from build123d import *

# Parameters (mm, degrees)
SKETCH_1_R                = 2.5
EXTRUDE_1_DEPTH           = 25.88
EXTRUDE_START             = 3
SKETCH_2_R                = 1
EXTRUDE_2_DEPTH           = 2
CUT_EXTRUDE_1_DEPTH       = 4
CUT_EXTRUDE_START         = 21.88
CUT_EXTRUDE_2_DEPTH       = 4
SKETCH_6_R                = 0.25
CUT_EXTRUDE_3_DEPTH       = 0.25
CUT_EXTRUDE_START_2       = 4.25
SKETCH_7_R                = 0.25
CUT_EXTRUDE_4_DEPTH       = 0.25
EXTRUDE_START_2           = 8
SKETCH_17_R               = 3.5
EXTRUDE_5_DEPTH           = 9.88
SKETCH_18_R               = 1
CUT_EXTRUDE_11_DEPTH      = 10
CUT_EXTRUDE_START_3       = 15.88
SKETCH_19_R               = 1
CUT_EXTRUDE_12_DEPTH      = 10
CUT_EXTRUDE_13_DEPTH      = 2.5
CUT_EXTRUDE_13_DEPTH_BACK = 2.5
SKETCH_20_W               = 4
SKETCH_20_H               = 1.6
CUT_EXTRUDE_14_DEPTH      = 28.789825476
CUT_EXTRUDE_14_DEPTH_BACK = 28.789825476
SKETCH_21_W               = 1.5
SKETCH_21_H               = 9.88
SKETCH_22_W               = 4
SKETCH_22_H               = 1.5
CUT_EXTRUDE_15_DEPTH      = 28.789825476


with BuildPart() as part:
    # 草图1 → 凸台-拉伸1 (new body)
    with BuildSketch(Plane(origin=(0, 0, 0), x_dir=(1, 0, 0), z_dir=(0, 1, 0))):
        with Locations(Location((0, 0, 0), (0, 0, 270))):
            Circle(SKETCH_1_R)
    extrude(amount=EXTRUDE_1_DEPTH)

    # 草图2 → 凸台-拉伸2 (add)
    with BuildSketch(Plane(origin=(0, 0, 0), x_dir=(1, 0, 0), z_dir=(0, 1, 0)).offset(EXTRUDE_START)):
        with BuildLine():
            Line((0.166666667, 2.494438258), (7.633333333, 1.995550606))
            ThreePointArc((7.633333333, 1.995550606), (9.5, 0), (7.633333333, -1.995550606))
            Line((7.633333333, -1.995550606), (0.166666667, -2.494438258))
            ThreePointArc((0.166666667, -2.494438258), (-2.5, 0), (0.166666667, 2.494438258))
        make_face()
        with Locations(Location((7.5, 0, 0), (0, 0, 270))):
            Circle(SKETCH_2_R, mode=Mode.SUBTRACT)
    extrude(amount=EXTRUDE_2_DEPTH)

    # 草图3 → 切除-拉伸1 (cut)
    with BuildSketch(Plane(origin=(0, 0, 0), x_dir=(1, 0, 0), z_dir=(0, 1, 0))):
        with BuildLine():
            Line((-1.854049622, -0.75), (-0.75, -0.75))
            Line((-0.75, -0.75), (-0.75, -1.854049622))
            ThreePointArc((-0.75, -1.854049622), (0, -2), (0.75, -1.854049622))
            Line((0.75, -1.854049622), (0.75, -0.75))
            Line((0.75, -0.75), (1.854049622, -0.75))
            ThreePointArc((1.854049622, -0.75), (2, 0), (1.854049622, 0.75))
            Line((1.854049622, 0.75), (0.75, 0.75))
            Line((0.75, 0.75), (0.75, 1.854049622))
            ThreePointArc((0.75, 1.854049622), (0, 2), (-0.75, 1.854049622))
            Line((-0.75, 1.854049622), (-0.75, 0.75))
            Line((-0.75, 0.75), (-1.854049622, 0.75))
            ThreePointArc((-1.854049622, 0.75), (-2, 0), (-1.854049622, -0.75))
        make_face()
    extrude(amount=CUT_EXTRUDE_1_DEPTH, mode=Mode.SUBTRACT)

    # 草图5 → 切除-拉伸2 (cut)
    with BuildSketch(Plane(origin=(0, 0, 0), x_dir=(1, 0, 0), z_dir=(0, 1, 0)).offset(CUT_EXTRUDE_START)):
        with BuildLine():
            Line((1.854049622, 0.75), (0.75, 0.75))
            Line((0.75, 0.75), (0.75, 1.854049622))
            ThreePointArc((0.75, 1.854049622), (0, 2), (-0.75, 1.854049622))
            Line((-0.75, 1.854049622), (-0.75, 0.75))
            Line((-0.75, 0.75), (-1.854049622, 0.75))
            ThreePointArc((-1.854049622, 0.75), (-2, 0), (-1.854049622, -0.75))
            Line((-1.854049622, -0.75), (-0.75, -0.75))
            Line((-0.75, -0.75), (-0.75, -1.854049622))
            ThreePointArc((-0.75, -1.854049622), (0, -2), (0.75, -1.854049622))
            Line((0.75, -1.854049622), (0.75, -0.75))
            Line((0.75, -0.75), (1.854049622, -0.75))
            ThreePointArc((1.854049622, -0.75), (2, 0), (1.854049622, 0.75))
        make_face()
    extrude(amount=CUT_EXTRUDE_2_DEPTH, mode=Mode.SUBTRACT)

    # 草图6 → 切除-拉伸3 (cut)
    with BuildSketch(Plane(origin=(0, 0, 0), x_dir=(1, 0, 0), z_dir=(0, 1, 0)).offset(CUT_EXTRUDE_START)):
        with Locations(Location((0.75, 0, 0), (0, 0, 270))):
            Circle(SKETCH_6_R)
    extrude(amount=-CUT_EXTRUDE_3_DEPTH, mode=Mode.SUBTRACT)

    # 草图7 → 切除-拉伸4 (cut)
    with BuildSketch(Plane(origin=(0, 0, 0), x_dir=(1, 0, 0), z_dir=(0, 1, 0)).offset(CUT_EXTRUDE_START_2)):
        with Locations(Location((0.75, 0, 0), (0, 0, 270))):
            Circle(SKETCH_7_R)
    extrude(amount=-CUT_EXTRUDE_4_DEPTH, mode=Mode.SUBTRACT)

    # 草图17 → 凸台-拉伸5 (add)
    with BuildSketch(Plane(origin=(0, 0, 0), x_dir=(1, 0, 0), z_dir=(0, 1, 0)).offset(EXTRUDE_START_2)):
        with Locations(Location((0, 0, 0), (0, 0, 270))):
            Circle(SKETCH_17_R)
    extrude(amount=EXTRUDE_5_DEPTH)

    # 草图18 → 切除-拉伸11 (cut)
    with BuildSketch(Plane(origin=(0, 0, 0), x_dir=(1, 0, 0), z_dir=(0, 1, 0))):
        with Locations(Location((0, 0, 0), (0, 0, 270))):
            Circle(SKETCH_18_R)
    extrude(amount=CUT_EXTRUDE_11_DEPTH, mode=Mode.SUBTRACT)

    # 草图19 → 切除-拉伸12 (cut)
    with BuildSketch(Plane(origin=(0, 0, 0), x_dir=(1, 0, 0), z_dir=(0, 1, 0)).offset(CUT_EXTRUDE_START_3)):
        with Locations(Location((0, 0, 0), (0, 0, 270))):
            Circle(SKETCH_19_R)
    extrude(amount=CUT_EXTRUDE_12_DEPTH, mode=Mode.SUBTRACT)

    # 草图20 → 切除-拉伸13 (cut, two sides: drawn at the far end of the back side and taken through both)
    with BuildSketch(Plane.XY.offset(-CUT_EXTRUDE_13_DEPTH_BACK)):
        with Locations((0, 15.68)):
            Rectangle(SKETCH_20_W, SKETCH_20_H)
        with Locations((0, 10.2)):
            Rectangle(SKETCH_20_W, SKETCH_20_H)
    extrude(amount=CUT_EXTRUDE_13_DEPTH + CUT_EXTRUDE_13_DEPTH_BACK, mode=Mode.SUBTRACT)

    # 草图21 → 切除-拉伸14 (cut, two sides: drawn at the far end of the back side and taken through both)
    with BuildSketch(Plane.XY.offset(-CUT_EXTRUDE_14_DEPTH_BACK)):
        with Locations((2.75, 12.94)):
            Rectangle(SKETCH_21_W, SKETCH_21_H)
    extrude(amount=CUT_EXTRUDE_14_DEPTH + CUT_EXTRUDE_14_DEPTH_BACK, mode=Mode.SUBTRACT)

    # 草图22 → 切除-拉伸15 (cut, through all)
    with BuildSketch(Plane(origin=(0, 0, 0), x_dir=(0, 0, -1), z_dir=(1, 0, 0))):
        with Locations((0, 12.94)):
            Rectangle(SKETCH_22_W, SKETCH_22_H)
    extrude(amount=CUT_EXTRUDE_15_DEPTH, mode=Mode.SUBTRACT)


solid = part.part
Verification items for the finished model (mm, model axes). A direction names the side the tool comes from. Give positions to 0.01 mm unless a question says otherwise; leave off trailing zeros. Loops run counter-clockwise (first coordinate to the right, second up) from the corner with the lowest first, then second, coordinate; pieces in that order, holes last.
1) Sectioned sample at C-C, the plane x = 5. Enter the section's corners in (y, z).
2) Sectioned sample at D-D, the plane y = 11.5. Enter the section's corners in (x, z), then the cut area to 3 significant figures.
3) Draft check along Y on faces 1 (the cylindrical face through (0, 2, 2)), 2 (the flat face through (1, 13, -2)), 3 (the flat face through (5, 3, 0)), 4 (the flat face through (0, 13, 0)). Enter one of: pulls with the +Y half, pulls with the -Y half, needs draft (parallel to the pull), parting line crosses it, or undercut.
4) Set-up check for faces 5 (the flat face through (-1, 24, 0.75)), 6 (the flat face through (0, 10, 2.5)), 7 (the flat face through (-0.75, 2, -1)), 8 (the flat face through (2, 14, 0)), 9 (the cylindrical face through (9.5, 4, 0)): record each of +Z, -Z, +X, -X, +Y, -Y from which the full face is reachable in a straight line by a thin tool's end or side.
5) Sectioned sample at B-B, the plane y = 20.25. Enter the section's corners in (x, z), then the cut area to 3 significant figures.
6) Depth check by flat-ended pin: pin 1 Ø0.6 at (y, z) = (24, -1.5) entering from +X; pin 2 Ø1.5 at (x, z) = (7, -0.5) entering from -Y; pin 3 Ø1.2 at (y, z) = (24.5, 1) entering from +X. Enter the tip coordinate at first touch or a pass-through.
7) Thickness scan on line 1 along Y through (x, z) = (-1, -2); line 2 along Y through (x, z) = (0.5, 1.5); line 3 along X through (y, z) = (8.1, 0). Record the ranges inside material, lowest first.
Answers:
1. outline: (3, -2.17) - (5, -2.17) - (5, 2.17) - (3, 2.17) - close
2. outline: (2, -2.87) - (2, 2.87) arc R3.5 ccw (long way) to start
2. area: 32.4 mm2
3. face 1: needs draft
3. face 2: undercut
3. face 3: pulls with the -Y half
3. face 4: undercut
4. face 5: +Y
4. face 6: +X
4. face 7: -Y
4. face 8: +Z, -Z, +X
4. face 9: +X, +Y, -Y
5. outline: circle Ø5 at (0, 0); hole circle Ø2 at (0, 0)
5. area: 16.5 mm2
6. pin 1: stops at x = 2.19
6. pin 2: stops at y = 3
6. pin 3: stops at x = 2.47
7. line 1: y = 0 to 9.4, 11 to 14.88, 16.48 to 25.88
7. line 2: y = 4 to 9.4, 11 to 12.19, 13.69 to 14.88, 16.48 to 21.88
7. line 3: x = -3.5 to -1, 1 to 2
